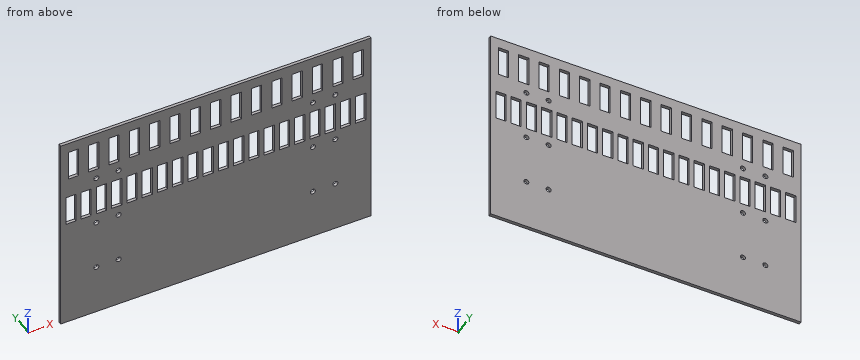
```python
from build123d import *

# Parameters (mm, degrees)
F0_W     = 305
F0_H     = 200
F0_R     = 2.5
F0_W_2   = 10
F0_H_2   = 30
F1_DEPTH = 3


with BuildPart() as f1:
    # F0 (on Front) → F1 (new body)
    with BuildSketch(Plane.XZ):
        Rectangle(F0_W, F0_H)
        with Locations((-117.5, -50)):
            Circle(F0_R, mode=Mode.SUBTRACT)
        with Locations((-95.5, -50)):
            Circle(F0_R, mode=Mode.SUBTRACT)
        with Locations((95.5, -50)):
            Circle(F0_R, mode=Mode.SUBTRACT)
        with Locations((117.5, -50)):
            Circle(F0_R, mode=Mode.SUBTRACT)
        with Locations((-117.5, 0)):
            Circle(F0_R, mode=Mode.SUBTRACT)
        with Locations((-95.5, 0)):
            Circle(F0_R, mode=Mode.SUBTRACT)
        with Locations((-142.5, 25)):
            Rectangle(F0_W_2, F0_H_2, mode=Mode.SUBTRACT)
        with Locations((-127.5, 25)):
            Rectangle(F0_W_2, F0_H_2, mode=Mode.SUBTRACT)
        with Locations((-112.5, 25)):
            Rectangle(F0_W_2, F0_H_2, mode=Mode.SUBTRACT)
        with Locations((-97.5, 25)):
            Rectangle(F0_W_2, F0_H_2, mode=Mode.SUBTRACT)
        with Locations((-82.5, 25)):
            Rectangle(F0_W_2, F0_H_2, mode=Mode.SUBTRACT)
        with Locations((-67.5, 25)):
            Rectangle(F0_W_2, F0_H_2, mode=Mode.SUBTRACT)
        with Locations((-52.5, 25)):
            Rectangle(F0_W_2, F0_H_2, mode=Mode.SUBTRACT)
        with Locations((-37.5, 25)):
            Rectangle(F0_W_2, F0_H_2, mode=Mode.SUBTRACT)
        with Locations((-22.5, 25)):
            Rectangle(F0_W_2, F0_H_2, mode=Mode.SUBTRACT)
        with Locations((-7.5, 25)):
            Rectangle(F0_W_2, F0_H_2, mode=Mode.SUBTRACT)
        with Locations((-117.5, 50)):
            Circle(F0_R, mode=Mode.SUBTRACT)
        with Locations((-95.5, 50)):
            Circle(F0_R, mode=Mode.SUBTRACT)
        with Locations((-140, 75)):
            Rectangle(F0_W_2, F0_H_2, mode=Mode.SUBTRACT)
        with Locations((-120, 75)):
            Rectangle(F0_W_2, F0_H_2, mode=Mode.SUBTRACT)
        with Locations((-100, 75)):
            Rectangle(F0_W_2, F0_H_2, mode=Mode.SUBTRACT)
        with Locations((-80, 75)):
            Rectangle(F0_W_2, F0_H_2, mode=Mode.SUBTRACT)
        with Locations((-60, 75)):
            Rectangle(F0_W_2, F0_H_2, mode=Mode.SUBTRACT)
        with Locations((-40, 75)):
            Rectangle(F0_W_2, F0_H_2, mode=Mode.SUBTRACT)
        with Locations((-20, 75)):
            Rectangle(F0_W_2, F0_H_2, mode=Mode.SUBTRACT)
        with Locations((7.5, 25)):
            Rectangle(F0_W_2, F0_H_2, mode=Mode.SUBTRACT)
        with Locations((22.5, 25)):
            Rectangle(F0_W_2, F0_H_2, mode=Mode.SUBTRACT)
        with Locations((37.5, 25)):
            Rectangle(F0_W_2, F0_H_2, mode=Mode.SUBTRACT)
        with Locations((52.5, 25)):
            Rectangle(F0_W_2, F0_H_2, mode=Mode.SUBTRACT)
        with Locations((67.5, 25)):
            Rectangle(F0_W_2, F0_H_2, mode=Mode.SUBTRACT)
        with Locations((95.5, 0)):
            Circle(F0_R, mode=Mode.SUBTRACT)
        with Locations((117.5, 0)):
            Circle(F0_R, mode=Mode.SUBTRACT)
        with Locations((82.5, 25)):
            Rectangle(F0_W_2, F0_H_2, mode=Mode.SUBTRACT)
        with Locations((97.5, 25)):
            Rectangle(F0_W_2, F0_H_2, mode=Mode.SUBTRACT)
        with Locations((112.5, 25)):
            Rectangle(F0_W_2, F0_H_2, mode=Mode.SUBTRACT)
        with Locations((127.5, 25)):
            Rectangle(F0_W_2, F0_H_2, mode=Mode.SUBTRACT)
        with Locations((142.5, 25)):
            Rectangle(F0_W_2, F0_H_2, mode=Mode.SUBTRACT)
        with Locations((0, 75)):
            Rectangle(F0_W_2, F0_H_2, mode=Mode.SUBTRACT)
        with Locations((20, 75)):
            Rectangle(F0_W_2, F0_H_2, mode=Mode.SUBTRACT)
        with Locations((40, 75)):
            Rectangle(F0_W_2, F0_H_2, mode=Mode.SUBTRACT)
        with Locations((60, 75)):
            Rectangle(F0_W_2, F0_H_2, mode=Mode.SUBTRACT)
        with Locations((95.5, 50)):
            Circle(F0_R, mode=Mode.SUBTRACT)
        with Locations((117.5, 50)):
            Circle(F0_R, mode=Mode.SUBTRACT)
        with Locations((80, 75)):
            Rectangle(F0_W_2, F0_H_2, mode=Mode.SUBTRACT)
        with Locations((100, 75)):
            Rectangle(F0_W_2, F0_H_2, mode=Mode.SUBTRACT)
        with Locations((120, 75)):
            Rectangle(F0_W_2, F0_H_2, mode=Mode.SUBTRACT)
        with Locations((140, 75)):
            Rectangle(F0_W_2, F0_H_2, mode=Mode.SUBTRACT)
    extrude(amount=F1_DEPTH)


solid = f1.part
```
The listing builds one solid part. Answer for the finished solid, in the listing's coordinates (mm). Round coordinates to 2 decimals unless told otherwise and drop trailing zeros. Loops run counter-clockwise (first coordinate to the right, second up) from the corner with the lowest first, then second, coordinate; pieces in that order, holes last.
Q1. Find the intervals of material crossed by line 1 (Z direction, x = -80.5, y = -0.6); line 2 (Z direction, x = -114, y = -2.45); line 3 (Z direction, x = 0, y = -2.3), in increasing order.
Q2. Section B-B, the plane x = 111 is taken. Determine the outline of the cut face in (y, z).
Q3. Section C-C, the plane z = 78 is taken. Count the separate pieces of the cut face and the enclosed holes in it, then the cut area to 3 significant figures.
Q4. Section A-A, the plane x = -39 is taken. Determine the outline of the cut face in (y, z).
Completed:
1. line 1: z = -100 to 10, 40 to 60, 90 to 100
1. line 2: z = -100 to 10, 40 to 100
1. line 3: z = -100 to 60, 90 to 100
2. outline: (-3, -100) - (0, -100) - (0, 10) - (-3, 10) - close; (-3, 40) - (0, 40) - (0, 100) - (-3, 100) - close
3. separate pieces: 16
3. enclosed holes: 0
3. area: 465 mm2
4. outline: (-3, -100) - (0, -100) - (0, 10) - (-3, 10) - close; (-3, 40) - (0, 40) - (0, 60) - (-3, 60) - close; (-3, 90) - (0, 90) - (0, 100) - (-3, 100) - close
